Here's how the part is built. I have some questions about the finished solid (model axes, mm). A direction names the side the tool comes from. Give positions to 0.01 mm unless a question says otherwise; leave off trailing zeros. Order: outer loops, then holes, each group sorted by start corner. A loop starts at its lowest first (then second) coordinate and runs counter-clockwise, first axis right, second up.
Autodesk Inventor part; units mm, degrees
ref_plane "YZ Plane" through (0, 0, 0) normal (1, 0, 0) x (0, 1, 0)
ref_plane "XZ Plane" through (0, 0, 0) normal (0, 1, 0) x (-1, 0, 0)
ref_plane "XY Plane" through (0, 0, 0) normal (0, 0, 1) x (1, 0, 0)
sketch "Sketch1" plane through (0, 0, 0) normal (0, 1, 0) x (-1, 0, 0)
  line L0 (-17.25, 26.25) -> (17.25, 26.25)
  line L1 (17.25, 26.25) -> (17.25, -26.25)
  line L2 (17.25, -26.25) -> (-17.25, -26.25)
  line L3 (-17.25, -26.25) -> (-17.25, 26.25)
  line L4 (-17.25, 26.25) -> (17.25, -26.25) construction
  line L5 (17.25, 26.25) -> (-17.25, -26.25) construction
  line L6 (17.25, -26.25) -> (-17.25, -26.25)
  line L7 (-17.25, -26.25) -> (-17.25, -76.25)
  line L8 (-17.25, -76.25) -> (17.25, -76.25)
  line L9 (17.25, -76.25) -> (17.25, -26.25)
  arc A0 (-17.25, -76.25) -> (17.25, -76.25) centre (0, -76.25) ccw
  point P0 (0, 0)
  dimension "d0" = 34.5
  dimension "d1" = 52.5
  dimension "d4" = 50
extrude "Floor" add sketch "Sketch1" along normal blind 10
sketch "Sketch3" plane through (0, 10, 0) normal (0, 1, 0) x (1, 0, 0)
  arc A0 (17.25, 76.25) -> (-17.25, 76.25) centre (0, 76.25) ccw
  circle A1 centre (0, 68.95) radius 10.25
  circle A2 centre (0, 68.95) radius 12.75
  line L0 (14.75, -23.75) -> (-14.75, -23.75)
  line L1 (-14.75, -23.75) -> (-14.75, 23.75)
  line L2 (-14.75, 23.75) -> (14.75, 23.75)
  line L3 (14.75, 23.75) -> (14.75, -23.75)
  line L4 (14.75, -23.75) -> (-14.75, 23.75) construction
  line L5 (-14.75, -23.75) -> (14.75, 23.75) construction
  line L6 (17.25, 26.25) -> (-17.25, 26.25)
  line L7 (-17.25, 26.25) -> (-17.25, -26.25)
  line L8 (-17.25, -26.25) -> (17.25, -26.25)
  line L9 (17.25, -26.25) -> (17.25, 26.25)
  line L10 (17.25, 26.25) -> (-17.25, -26.25) construction
  line L11 (-17.25, 26.25) -> (17.25, -26.25) construction
  line L12 (0, 23.75) -> (0, 68.95)
  point P0 (0, 0)
  dimension "d14" = 20.5
  dimension "d18" = 29.5
  dimension "d19" = 47.5
  dimension "d38" = 45.2
  dimension "d54" = 25.5
extrude "Slots" add sketch "Sketch3" along normal blind 34
sketch "Sketch4" plane through (17.25, 0, 26.25) normal (1, 0, 0) x (0, 0, -1)
  line L0 (2.5, 10) -> (50, 10)
  line L1 (50, 10) -> (50, 44)
  line L2 (50, 44) -> (2.5, 44)
  line L3 (2.5, 44) -> (2.5, 10)
  line L4 (26.25, 10) -> (38.25, 10)
  line L5 (2.5, 10) -> (50, 10)
  line L6 (38.25, 10) -> (14.25, 10)
  line L7 (10.75, 33) -> (34.75, 33)
  line L8 (34.75, 33) -> (34.75, 21)
  line L9 (34.75, 21) -> (10.75, 21)
  line L10 (10.75, 21) -> (10.75, 33)
  line L11 (10.75, 33) -> (34.75, 21) construction
  line L12 (34.75, 33) -> (10.75, 21) construction
  circle A0 centre (10.75, 33) radius 1.35
  circle A1 centre (34.75, 33) radius 1.35
  circle A2 centre (34.75, 21) radius 1.35
  circle A3 centre (10.75, 21) radius 1.35
  line L13 (50, 10) -> (50, 44)
  line L14 (50, 27) -> (34.75, 27)
  line L15 (34.75, 27) -> (22.75, 27)
  point P0 (26.25, 0)
  point P1 (22.75, 27)
  dimension "d24" = 12
  dimension "d25" = 24
  dimension "d26" = 2.7
  dimension "d27" = 2.7
  dimension "d28" = 2.7
  dimension "d29" = 2.7
  dimension "d56" = 15.25
  dimension "d57" = 12
extrude "Screws/Sides" cut sketch "Sketch4" against normal through all contours A1 L7 L8 | L8 L7 A1 | A2 L9 L8 | L8 L9 A2 | A0 L10 L7 | L7 L10 A0 | A3 L10 L9 | L9 L10 A3
sketch "Sketch5" plane through (0, 44, 0) normal (0, 1, 0) x (1, 0, 0)
  line L0 (14.75, -21.75) -> (-14.75, -21.75)
  line L1 (-14.75, -21.75) -> (-14.75, 21.75)
  line L2 (-14.75, 21.75) -> (14.75, 21.75)
  line L3 (14.75, 21.75) -> (14.75, -21.75)
  line L4 (14.75, -21.75) -> (-14.75, 21.75) construction
  line L5 (-14.75, -21.75) -> (14.75, 21.75) construction
  line L6 (12.75, 23.75) -> (-12.75, 23.75)
  line L7 (-12.75, 23.75) -> (-12.75, -23.75)
  line L8 (-12.75, -23.75) -> (12.75, -23.75)
  line L9 (12.75, -23.75) -> (12.75, 23.75)
  line L10 (12.75, 23.75) -> (-12.75, -23.75) construction
  line L11 (-12.75, 23.75) -> (12.75, -23.75) construction
  line L12 (-12.75, 21.75) -> (-14.75, 21.75)
  line L13 (12.75, 23.75) -> (12.75, 21.75)
  line L14 (12.75, -21.75) -> (14.75, -21.75)
  line L15 (12.75, -23.75) -> (12.75, -21.75)
  line L16 (-14.75, -21.75) -> (-14.75, -23.75)
  line L17 (-14.75, -23.75) -> (-12.75, -23.75)
  line L18 (-14.75, -21.75) -> (-12.75, -23.75)
  line L19 (-14.75, -23.75) -> (-14.75, -21.75)
  line L20 (-14.75, 21.75) -> (-12.75, 23.75)
  line L21 (-14.75, 23.75) -> (-14.75, 21.75)
  line L22 (-14.75, -23.75) -> (-14.75, 23.75)
  line L23 (12.75, 23.75) -> (14.75, 23.75)
  line L24 (14.75, 23.75) -> (14.75, 21.75)
  line L25 (12.75, 23.75) -> (14.75, 21.75)
  line L26 (14.75, 23.75) -> (12.75, 23.75)
  line L27 (14.75, -23.75) -> (12.75, -23.75)
  line L28 (14.75, -23.75) -> (-14.75, -23.75)
  line L29 (14.75, -21.75) -> (12.75, -23.75)
  line L30 (14.75, -23.75) -> (14.75, -21.75)
  line L31 (14.75, 23.75) -> (14.75, -23.75)
  line L32 (-14.75, 23.75) -> (-12.75, 23.75)
  line L33 (14.75, 23.75) -> (-14.75, 23.75)
  point P0 (0, 0)
  dimension "d32" = 43.5
  dimension "d33" = 25.5
extrude "Servo Corners" add sketch "Sketch5" against normal blind 34 contours L30 L27 L29 | L25 L23 L24 | L17 L16 L18 | L20 L21 L32
sketch "Sketch6" plane through (0, 44, 0) normal (0, 1, 0) x (1, 0, 0)
  line L0 (-12.75, 23.75) -> (12.75, 23.75)
  line L1 (0, 23.75) -> (0, 12.5)
  circle A0 centre (0, 68.95) radius 10.25
  line L2 (0, 12.5) -> (0, 68.95)
  point P0 (0, 0)
  dimension "d36" = 11.25
  dimension "d37" = 56.45
sketch "Sketch7" plane through (-17.25, 0, 26.25) normal (0, 0, 1) x (1, 0, 0)
  line L0 (0, 0) -> (34.5, 0)
  line L1 (34.5, 0) -> (34.5, 44)
  line L2 (34.5, 44) -> (0, 44)
  line L3 (0, 44) -> (0, 0)
  point P0 (17.25, 0)
extrude "Mount Extension" add sketch "Sketch7" along normal blind 30
sketch "Sketch8" plane through (-17.25, 0, 56.25) normal (0, 0, 1) x (1, 0, 0)
  line L0 (17.25, 0) -> (17.25, 10)
  line L1 (30, 44) -> (4.5, 44)
  line L2 (17.25, 27) -> (17.25, 35.5)
  line L3 (34.5, 10) -> (34.5, 44)
  line L4 (0, 10) -> (0, 44)
  line L5 (17.25, 35.5) -> (8.625, 35.5)
  circle A0 centre (8.625, 35.5) radius 2.6035
  line L6 (17.25, 10) -> (8.625, 10)
  line L7 (30, 10) -> (4.5, 10)
  line L8 (8.625, 10) -> (8.625, 18.5)
  circle A1 centre (8.625, 18.5) radius 2.6035
  line L9 (34.5, 35.5) -> (25.875, 35.5)
  dimension "d41" = 10
  dimension "d42" = 5.207
  dimension "d43" = 8.5
  dimension "d44" = 5.207
  dimension "d47" = 8.625
extrude "Mount Holes" cut sketch "Sketch8" against normal blind 20
pattern_linear "Rectangular Pattern1" count 2 spacing 17.25 along (1, 0, 0) of "Mount Holes"
sketch "Sketch11" plane through (17.25, 0, -76.25) normal (1, 0, 0) x (0, 0, -1)
  line L0 (-84.55, 10) -> (-71.55, 10)
  line L1 (-71.55, 10) -> (-71.55, 18.5)
  line L2 (-71.55, 18.5) -> (-84.55, 18.5)
  line L3 (-84.55, 18.5) -> (-84.55, 10)
  circle A0 centre (-67.75, 21) radius 1.35
  line L4 (-67.75, 21) -> (-67.75, 10)
  line L5 (-98, 10) -> (-54.5, 10)
  line L6 (-67.75, 10) -> (-71.55, 10)
  point P0 (-76.25, 0)
  dimension "d58" = 13
  dimension "d59" = 8.5
  dimension "d60" = 3.8
extrude "Wiring Holes" cut sketch "Sketch11" against normal through all contours L3 L2 L1 L0
sketch "Sketch12" plane through (0, 44, 0) normal (0, 1, 0) x (1, 0, 0)
  line L0 (14.75, -23.75) -> (-14.75, -23.75)
  line L1 (-14.75, -23.75) -> (-14.75, 23.75)
  line L2 (-14.75, 23.75) -> (14.75, 23.75)
  line L3 (14.75, 23.75) -> (14.75, -23.75)
  line L4 (14.75, -23.75) -> (-14.75, 23.75) construction
  line L5 (-14.75, -23.75) -> (14.75, 23.75) construction
  point P0 (0, 0)
  dimension "d63" = 29.5
  dimension "d64" = 47.5
properties part number "JointBase3DPrint"
Q1. If we section it at A-A on z = 15.5: List the corners of the cut face in (x, y) for me.
Filled sheet:
outline: (-17.25, 0) - (17.25, 0) - (17.25, 19.65) - (14.75, 19.65) - (14.75, 10) - (-14.75, 10) - (-14.75, 19.65) - (-17.25, 19.65) - close; (-17.25, 22.35) - (-14.75, 22.35) - (-14.75, 31.65) - (-17.25, 31.65) - close; (-17.25, 34.35) - (-14.75, 34.35) - (-14.75, 44) - (-17.25, 44) - close; (14.75, 22.35) - (17.25, 22.35) - (17.25, 31.65) - (14.75, 31.65) - close; (14.75, 34.35) - (17.25, 34.35) - (17.25, 44) - (14.75, 44) - close
Q2. Thinking about a two-plate mould opening in X: for faces 1 (the face through (-1.66, 26.76, -56.31)), 2 (the face through (-16, 14, 8.3)), 3 (the face through (0, 10, 0)), which applies, released by +X, released by -X, zero draft, split by the parting line, or undercut?
Filled sheet:
face 1: split by the parting line
face 2: zero draft
face 3: undercut
Q3. If we section it at C-C on x = 4: List the corners of the cut face in (y, z) for me, plus the area to 3 significant figures.
Filled sheet:
outline: (0, -93.03) - (10, -93.03) - (10, -81.06) - (44, -81.06) - (44, -78.39) - (10, -78.39) - (10, -59.51) - (44, -59.51) - (44, -56.84) - (10, -56.84) - (10, -26.25) - (44, -26.25) - (44, -23.75) - (10, -23.75) - (10, 23.75) - (44, 23.75) - (44, 56.25) - (0, 56.25) - close
area: 2,860 mm2
Q4. If we section it at D-D on z = -68.95: List the corners of the cut face in (x, y) for me.
Filled sheet:
outline: (-17.25, 0) - (17.25, 0) - (17.25, 10) - (12.75, 10) - (12.75, 44) - (10.25, 44) - (10.25, 10) - (-10.25, 10) - (-10.25, 44) - (-12.75, 44) - (-12.75, 10) - (-17.25, 10) - close
Q5. I need wall thicknesses on L1, parallel to Y at x = 16.75, z = -8.5; L2, parallel to Z at x = 15.7, y = 33; L3, parallel to X at y = 18.5, z = 48.5. Which ranges of each line are inside material? Lowest first, please.
Filled sheet:
L1: y = 0 to 19.65, 22.35 to 31.65, 34.35 to 44
L2: z = -26.25 to -9.85, -7.15 to 14.15, 16.85 to 56.25
L3: x = -17.25 to -11.23, -6.02 to 6.02, 11.23 to 17.25
Q6. If we section it at B-B on z = 38: Give the number of separate pieces and of enclosed holes in the cut face, plus the area to 3 significant figures.
Filled sheet:
separate pieces: 1
enclosed holes: 4
area: 1,430 mm2
Q7. I'm going to push flat-ended pins straight in: P1, Ø8.5, axis at x = 8.625, y = 35.5, coming from the -Z side; P2, Ø2, axis at x = 11, z = -43.5, coming from the +Y side; P3, Ø2.5, axis at y = 33, z = 15.5, coming from the +X side; P4, Ø1.6, axis at x = 9, y = 17.5, coming from the +Z side. Where does each tip first touch, or does it pass through?
Filled sheet:
P1: stops at z = -80.93
P2: stops at y = 10
P3: passes through
P4: stops at z = 36.25
Q8. For faces 4 (the face through (0, 44, 33)), 5 (the face through (0, 22, 56.25)), 6 (the face through (-9, 36, 36.25)), 7 (the face through (-16, 14, -4.7)), 8 (the face through (-1.334, 26.762, -58.787)), which set-ups out of +Z, -Z, +X, -X, +Y, -Y let a thin tool reach every point of the face, with its end or its side?
Filled sheet:
face 4: +Z, -Z, +X, -X, +Y
face 5: +Z, +X, -X, +Y, -Y
face 6: +Z
face 7: +X, -X
face 8: +Y
